```python
from build123d import *

# Parameters (mm, degrees)
SKETCH_1_W          = 60
SKETCH_1_H          = 89.5
SKETCH_1_R          = 1.6
EXTRUDE_1_DEPTH     = 1
CUT_EXTRUDE_1_DEPTH = 10
FILLET_1_R          = 2
SKETCH_3_W          = 9
SKETCH_3_H          = 10
CUT_EXTRUDE_2_DEPTH = 10
FILLET_2_R          = 1


with BuildPart() as part:
    # 草图1 → 凸台-拉伸1 (new body)
    with BuildSketch(Plane.XY):
        Rectangle(SKETCH_1_W, SKETCH_1_H)
        with Locations((27, 14.75)):
            Circle(SKETCH_1_R, mode=Mode.SUBTRACT)
        with Locations((27, -5.25)):
            Circle(SKETCH_1_R, mode=Mode.SUBTRACT)
    extrude(amount=EXTRUDE_1_DEPTH)

    # 草图2 → 切除-拉伸1 (cut)
    with BuildSketch(Plane.XY.offset(1)):
        with BuildLine():
            Line((-24.45, 32.5), (-24.45, 17.5))
            ThreePointArc((-24.45, 17.5), (-26, 15.95), (-27.55, 17.5))
            Line((-27.55, 17.5), (-27.55, 32.5))
            ThreePointArc((-27.55, 32.5), (-26, 34.05), (-24.45, 32.5))
        make_face()
        with BuildLine():
            Line((-24.45, -17.5), (-24.45, -32.5))
            ThreePointArc((-24.45, -32.5), (-26, -34.05), (-27.55, -32.5))
            Line((-27.55, -32.5), (-27.55, -17.5))
            ThreePointArc((-27.55, -17.5), (-26, -15.95), (-24.45, -17.5))
        make_face()
    extrude(amount=-CUT_EXTRUDE_1_DEPTH, mode=Mode.SUBTRACT)

    # 圆角1
    fillet_1_edges = [part.edges().sort_by_distance(p)[0] for p in [
        (30, -44.75, 0.5),
        (-30, -44.75, 0.5),
        (-30, 44.75, 0.5),
        (30, 44.75, 0.5),
    ]]
    fillet(fillet_1_edges, radius=FILLET_1_R)

    # 草图3 → 切除-拉伸2 (cut)
    with BuildSketch(Plane(origin=(0, 0, 0), x_dir=(-1, 0, 0), z_dir=(0, 0, -1))):
        with Locations((-20, -44.75)):
            Rectangle(SKETCH_3_W, SKETCH_3_H)
    extrude(amount=-CUT_EXTRUDE_2_DEPTH, mode=Mode.SUBTRACT)

    # 圆角2
    fillet_2_edges = [part.edges().sort_by_distance(p)[0] for p in [
        (24.5, -44.75, 0.5),
        (15.5, -44.75, 0.5),
        (24.5, -39.75, 0.5),
        (15.5, -39.75, 0.5),
    ]]
    fillet(fillet_2_edges, radius=FILLET_2_R)


solid = part.part
```
For this review, take the finished solid that the model builds, in its own axes (mm). Give positions to 0.01 mm unless a question says otherwise; leave off trailing zeros. Loops run counter-clockwise (first coordinate to the right, second up) from the corner with the lowest first, then second, coordinate; pieces in that order, holes last. Notation, with made-up numbers: M 85,-11.75 L 131,-11.75 A27 ccw 131,24.25 Z; hole C -7,-32 d7. An arc over 180 degrees is marked long. One line per item, written item: value. Start each with the question number.
Q1. Add section A-A (y = -31.5). Give the boundary of the cut face in (x, z), and give its area (3 significant figures).
Q2. Add section C-C (z = 0.6). Give the boundary of the cut face in (x, y), and give its area (3 significant figures).
Q3. Draft analysis for pull direction Y (two halves, no side actions). For faces 1 (the face through (25.82, 15.83, 0.49)), 2 (the face through (29.4, 44.18, 0.51)), 3 (the face through (25.82, -4.17, 0.49)), 4 (the face through (-29.43, -44.15, 0.51)), state which applies: released by +Y, released by -Y, zero draft, split by the parting line, or undercut.
Q4. Clearance check with a flat-ended pin moving along its axis: pin 1 Ø3 at (x, y) = (27, 14.75) entering from -Z. State where the tip first meets the part, or that it passes through.
Q5. Add section D-D (x = 21.5). Give the boundary of the cut face in (y, z).
Q6. Add section B-B (x = -26). Give the boundary of the cut face in (y, z), and give its area (3 significant figures).
Q7. For L1, parallel to Y at x = 27, z = 0.2; L2, parallel to X at y = 22.5, z = 0.7; L3, parallel to X at y = -4, z = 0.5, list the stretches that pass through material, from the lowest coordinate up.
Reply:
1. outline: M -30,0 L -27.55,0 L -27.55,1 L -30,1 Z; M -24.45,0 L 30,0 L 30,1 L -24.45,1 Z
1. area: 56.9 mm²
2. outline: M -30,-42.75 A2 ccw -28,-44.75 L 14.5,-44.75 A1 ccw 15.5,-43.75 L 15.5,-40.75 A1 cw 16.5,-39.75 L 23.5,-39.75 A1 cw 24.5,-40.75 L 24.5,-43.75 A1 ccw 25.5,-44.75 L 28,-44.75 A2 ccw 30,-42.75 L 30,42.75 A2 ccw 28,44.75 L -28,44.75 A2 ccw -30,42.75 Z; hole M -27.55,-32.5 A1.55 ccw -24.45,-32.5 L -24.45,-17.5 A1.55 ccw -27.55,-17.5 Z; hole M -27.55,17.5 A1.55 ccw -24.45,17.5 L -24.45,32.5 A1.55 ccw -27.55,32.5 Z; hole C 27,-5.25 d3.2; hole C 27,14.75 d3.2
2. area: 5,200 mm²
3. face 1: undercut
3. face 2: released by +Y
3. face 3: undercut
3. face 4: released by -Y
4. pin 1: through
5. outline: M -39.75,0 L 44.75,0 L 44.75,1 L -39.75,1 Z
6. outline: M -44.75,0 L -34.05,0 L -34.05,1 L -44.75,1 Z; M -15.95,0 L 15.95,0 L 15.95,1 L -15.95,1 Z; M 34.05,0 L 44.75,0 L 44.75,1 L 34.05,1 Z
6. area: 53.3 mm²
7. L1: -44.75 to -6.85, -3.65 to 13.15, 16.35 to 44.75
7. L2: -30 to -27.55, -24.45 to 30
7. L3: -30 to 26, 28 to 30
